Design review of the part built by this model. Coordinates are the model's own, in mm. A direction names the side the tool comes from. Coordinates: 2 decimals unless noted, no trailing zeros. Loops run counter-clockwise (first coordinate to the right, second up) from the corner with the lowest first, then second, coordinate; pieces in that order, holes last. Notation, with made-up numbers: M 79,11 L 115,11 A24 ccw 115,42 Z; hole C -26,-16 d5. An arc over 180 degrees is marked long. Write item = value, one per line. Start each with the question number.
from build123d import *

# Parameters (mm, degrees)
BOSS_EXTRUDE1_DEPTH = 10
SKETCH2_R           = 1.5
CUT_EXTRUDE1_DEPTH  = 38
CUT_EXTRUDE2_REACH  = 47.76
SKETCH3_R           = 2.5


with BuildPart() as part:
    # Sketch1 → Boss-Extrude1 (new body)
    with BuildSketch(Plane.XY):
        with BuildLine():
            Line((0, 0), (25, 0))
            Line((25, 0), (25, 5))
            Line((25, 5), (22, 5))
            Line((22, 5), (22, 3))
            Line((22, 3), (14, 3))
            Line((14, 3), (14, 5))
            Line((14, 5), (7, 5))
            ThreePointArc((7, 5), (5.585786438, 5.585786438), (5, 7))
            Line((5, 7), (5, 25.100505063))
            ThreePointArc((5, 25.100505063), (5.152240935, 25.865871928), (5.585786438, 26.514718626))
            Line((5.585786438, 26.514718626), (10.485281374, 31.414213562))
            ThreePointArc((10.485281374, 31.414213562), (11.134128072, 31.847759065), (11.899494937, 32))
            Line((11.899494937, 32), (14, 32))
            Line((14, 32), (14, 34))
            Line((14, 34), (22, 34))
            Line((22, 34), (22, 32))
            Line((22, 32), (25, 32))
            Line((25, 32), (25, 37))
            Line((25, 37), (9, 37))
            Line((9, 37), (0, 28))
            Line((0, 28), (0, 0))
        make_face()
    extrude(amount=BOSS_EXTRUDE1_DEPTH)

    # Sketch2 → Cut-Extrude1 (cut)
    with BuildSketch(Plane(origin=(0, 37, 0), x_dir=(1, 0, 0), z_dir=(0, 1, 0))):
        with Locations(Location((18, -5, 0), (0, 0, 270))):
            Circle(SKETCH2_R)
    extrude(amount=-CUT_EXTRUDE1_DEPTH, mode=Mode.SUBTRACT)

    # Sketch3 → Cut-Extrude2 (cut, up to next)
    with BuildSketch(Plane.ZY, mode=Mode.PRIVATE) as cut_extrude2_sk1:
        with Locations((5, 12)):
            Circle(SKETCH3_R)
    cut_extrude2_tool1 = extrude(cut_extrude2_sk1.sketch, amount=-CUT_EXTRUDE2_REACH, mode=Mode.PRIVATE) & part.part
    add(cut_extrude2_tool1.solids().sort_by_distance((0, 12, 5))[0], mode=Mode.SUBTRACT)


solid = part.part
Q1. Add section A-A on x = 18. State the section outline as (y, z) points.
Q2. To check wall thickness, follow line 1 (X direction, y = 4.5, z = 8.75); line 2 (Y direction, x = 16.25, z = 3); line 3 (Y direction, x = 12.5, z = 7.25). State the ranges of each line that lie inside material, in increasing order. Write a range as from..to.
Q3. Add section C-C on x = 15. State the section outline as (y, z) points, plus the area to 3 significant figures.
Q4. Add section B-B on y = 14. State the section outline as (x, z) points.
Q5. Mouldability with a two-part tool opening along Y and no side actions: class faces 1 (the face through (4, 19, 0)), 2 (the face through (15, 37, 5)), 3 (the face through (16, 34, 5)), 4 (the face through (11.12, 31.84, 4.93)) as released by +Y, released by -Y, zero draft, split by the parting line, or undercut.
Q6. Clearance check with flat-ended pins moving along their axes: P1, Ø5, axis at y = 20, z = 2, coming from the +X side; P2, Ø1, axis at y = 33, z = 7, coming from the -X side. State where each tip first meets the part, or that it passes through.
Q7. For faces 5 (the face through (2.46, 9.78, 6.15)), 6 (the face through (14, 4, 5)), 7 (the face through (13, 32, 5)), list the 3-axis set-ups (+Z, -Z, +X, -X, +Y, -Y) from which the entire face can be reached by the end or side of a thin tool; tool diameter is ignored.
Q8. Add section D-D on z = 4. Give the number of separate pieces and of enclosed holes in the cut face, plus the area to 3 significant figures.
Values follow:
q1.outline = M 0,0 L 3,0 L 3,3.5 L 0,3.5 Z; M 0,6.5 L 3,6.5 L 3,10 L 0,10 Z; M 34,0 L 37,0 L 37,3.5 L 34,3.5 Z; M 34,6.5 L 37,6.5 L 37,10 L 34,10 Z
q2.line_1 = 0..14, 22..25
q2.line_2 = 0..3, 34..37
q2.line_3 = 0..5, 32..37
q3.outline = M 0,0 L 3,0 L 3,10 L 0,10 Z; M 34,0 L 37,0 L 37,10 L 34,10 Z
q3.area = 60.0 mm2
q4.outline = M 0,0 L 5,0 L 5,3.5 L 0,3.5 Z; M 0,6.5 L 5,6.5 L 5,10 L 0,10 Z
q5.face_1 = zero draft
q5.face_2 = released by +Y
q5.face_3 = undercut
q5.face_4 = undercut
q6.P1 = 5
q6.P2 = 4.5
q7.face_5 = +X, -X
q7.face_6 = +Z, -Z
q7.face_7 = +Z, -Z, +X
q8.separate_pieces = 4
q8.enclosed_holes = 0
q8.area = 296 mm2
